```python
from build123d import *

# Parameters (mm, degrees)
SKETCH1_W            = 10
SKETCH1_H            = 50
SKETCH1_W_2          = 4
SKETCH1_H_2          = 30
BOSS_EXTRUDE1_DEPTH  = 2
SKETCH2_W            = 50
SKETCH2_H            = 10
SKETCH2_W_2          = 37
SKETCH2_H_2          = 5
BOSS_EXTRUDE2_DEPTH  = 12
SKETCH6_W            = 133.5
SKETCH6_H            = 10
SKETCH6_W_2          = 37
SKETCH6_H_2          = 5
BOSS_EXTRUDE7_DEPTH  = 2
SKETCH3_W            = 133.5
SKETCH3_H            = 10
BOSS_EXTRUDE3_DEPTH  = 5.7
SKETCH4_W            = 10.25
SKETCH4_H            = 10
BOSS_EXTRUDE4_DEPTH  = 10
CHAMFER1_SIZE        = 2
BOSS_EXTRUDE5_START  = -38
SKETCH5_W            = 10
SKETCH5_H            = 19
SKETCH5_R            = 2.2
BOSS_EXTRUDE5_DEPTH  = 2
BOSS_EXTRUDE6_START  = -24
SKETCH5_3_W          = 10
SKETCH5_3_H          = 22.4
SKETCH5_3_R          = 2
BOSS_EXTRUDE6_DEPTH  = 2
BOSS_EXTRUDE8_DEPTH  = 1
BOSS_EXTRUDE9_START  = -10
BOSS_EXTRUDE9_DEPTH  = 1
BOSS_EXTRUDE10_DEPTH = 1
BOSS_EXTRUDE11_START = -10
BOSS_EXTRUDE11_DEPTH = 1
BOSS_EXTRUDE12_START = -9.5
BOSS_EXTRUDE12_DEPTH = 10
BOSS_EXTRUDE13_DEPTH = 10
CHAMFER2_SIZE        = 10


with BuildPart() as part:
    # Sketch1 → Boss-Extrude1 (new body)
    with BuildSketch(Plane(origin=(0, 0, 0), x_dir=(0, 1, 0), z_dir=(0, 0, 1))):
        Rectangle(SKETCH1_W, SKETCH1_H)
        with Locations((-0.5, -3)):
            Rectangle(SKETCH1_W_2, SKETCH1_H_2, mode=Mode.SUBTRACT)
    extrude(amount=BOSS_EXTRUDE1_DEPTH)

    # Sketch2 → Boss-Extrude2 (add)
    with BuildSketch(Plane.XY.offset(2)):
        Rectangle(SKETCH2_W, SKETCH2_H)
        with Locations((3.5, -1)):
            Rectangle(SKETCH2_W_2, SKETCH2_H_2, mode=Mode.SUBTRACT)
    extrude(amount=BOSS_EXTRUDE2_DEPTH)

    # Sketch6 → Boss-Extrude7 (add)
    with BuildSketch(Plane.XY.offset(14)):
        with Locations((-41.75, 0)):
            Rectangle(SKETCH6_W, SKETCH6_H)
        with Locations((3.5, -1)):
            Rectangle(SKETCH6_W_2, SKETCH6_H_2, mode=Mode.SUBTRACT)
    extrude(amount=BOSS_EXTRUDE7_DEPTH)

    # Sketch3 → Boss-Extrude3 (add)
    with BuildSketch(Plane.XY.offset(16)):
        with Locations((-41.75, 0)):
            Rectangle(SKETCH3_W, SKETCH3_H)
        Polygon((22, -3.5), (-15, -3.5), (-15, -2), (-64.5, -2), (-64.5, 1.5), (22, 1.5), align=None, mode=Mode.SUBTRACT)
    extrude(amount=BOSS_EXTRUDE3_DEPTH)

    # Sketch4 → Boss-Extrude4 (add)
    with BuildSketch(Plane.XY.offset(21.7)):
        with Locations((-103.375, 0)):
            Rectangle(SKETCH4_W, SKETCH4_H)
        Polygon((-64.5, -2), (-64.5, 1.5), (-59.5, 1.5), (-59.5, 5), (-74.75, 5), (-74.75, -5), (25, -5), (25, 5), (1.7, 5), (1.7, 1.5), (22, 1.5), (22, -3.5), (-15, -3.5), (-15, -2), align=None)
    extrude(amount=BOSS_EXTRUDE4_DEPTH)

    # Chamfer1
    chamfer1_edges = [part.edges().sort_by_distance(p)[0] for p in [
        (-98.25, 0, 21.7),
        (-74.75, 0, 21.7),
    ]]
    chamfer(chamfer1_edges, length=CHAMFER1_SIZE)



with BuildPart() as body_2:
    # Sketch5 → Boss-Extrude5 (new body)
    with BuildSketch(Plane.XY.offset(31.7).offset(BOSS_EXTRUDE5_START)):
        with Locations((10.5, 14.5)):
            Rectangle(SKETCH5_W, SKETCH5_H)
        with Locations((10.5, 14.5)):
            Circle(SKETCH5_R, mode=Mode.SUBTRACT)
    extrude(amount=BOSS_EXTRUDE5_DEPTH)


with BuildPart() as body_3:
    # Sketch5<3> → Boss-Extrude6 (new body)
    with BuildSketch(Plane.XY.offset(31.7).offset(BOSS_EXTRUDE6_START)):
        with Locations((-103.5, 16.2)):
            Rectangle(SKETCH5_3_W, SKETCH5_3_H)
        with Locations((-103.5, 18.5)):
            Circle(SKETCH5_3_R, mode=Mode.SUBTRACT)
    extrude(amount=BOSS_EXTRUDE6_DEPTH)


with BuildPart() as part_1:
    add(part.part)

    add(body_2.part)  # Boss-Extrude8 merges body 2
    # Sketch7 → Boss-Extrude8 (add)
    with BuildSketch(Plane.YZ.offset(15.5)):
        Polygon((5, -4.3), (20, -4.3), (5, 7.7), align=None)
    extrude(amount=-BOSS_EXTRUDE8_DEPTH)

    # Sketch7<2> → Boss-Extrude9 (add)
    with BuildSketch(Plane.YZ.offset(15.5).offset(BOSS_EXTRUDE9_START)):
        Polygon((5, -4.3), (20, -4.3), (5, 7.7), align=None)
    extrude(amount=BOSS_EXTRUDE9_DEPTH)


    add(body_3.part)  # Boss-Extrude10 merges body 3
    # Sketch8 → Boss-Extrude10 (add)
    with BuildSketch(Plane.YZ.offset(-98.5)):
        Polygon((5, 9.7), (20, 9.7), (5, 21.7), align=None)
    extrude(amount=-BOSS_EXTRUDE10_DEPTH)

    # Sketch8<2> → Boss-Extrude11 (add)
    with BuildSketch(Plane.YZ.offset(-98.5).offset(BOSS_EXTRUDE11_START)):
        Polygon((5, 9.7), (20, 9.7), (5, 21.7), align=None)
    extrude(amount=BOSS_EXTRUDE11_DEPTH)

    # Sketch9 → Boss-Extrude12 (add)
    with BuildSketch(Plane.YZ.offset(25).offset(BOSS_EXTRUDE12_START)):
        Polygon((5, -6.3), (2, 0), (5, 0), align=None)
    extrude(amount=-BOSS_EXTRUDE12_DEPTH)

    # Sketch10 → Boss-Extrude13 (add)
    with BuildSketch(Plane.YZ.offset(-98.5)):
        Polygon((5, 7.7), (5, 14), (2, 14), align=None)
    extrude(amount=-BOSS_EXTRUDE13_DEPTH)

    # Chamfer2
    chamfer2_edges = [part_1.edges().sort_by_distance(p)[0] for p in [
        (-108.5, -5, 22.85),
    ]]
    chamfer(chamfer2_edges, length=CHAMFER2_SIZE)


solid = part_1.part
```
Design review of the part built by this model. Coordinates are the model's own, in mm. A direction names the side the tool comes from. Give positions to 0.01 mm unless a question says otherwise; leave off trailing zeros. Loops run counter-clockwise (first coordinate to the right, second up) from the corner with the lowest first, then second, coordinate; pieces in that order, holes last. Notation, with made-up numbers: M 51,3.25 L 70,3.25 A25 ccw 70,39.25 Z; hole C 62,-20 d6. An arc over 180 degrees is marked long. Return JSON: item names as keys, results as strings. Group by question number.
Item 1: We need section B-B (z = 12.5). Give the boundary of the cut face in (x, y), and give its area (3 significant figures).
Item 2: Insertion check: pin 1 Ø0.6 at (x, z) = (11, -5.5) entering from +Y; pin 2 Ø10 at (x, y) = (-66, 11.5) entering from -Z; pin 3 Ø15 at (x, z) = (6, 22) entering from +Y; pin 4 Ø8 at (x, y) = (-92, 5) entering from +Z. Each pin has a flat end and moves straight along its axis. Give the tip position at first contact, or say it passes through.
Item 3: For probe 1 along X at (y, z) = (7.5, 3.5); probe 2 along X at (y, z) = (-1, 12); probe 3 along Y at (x, z) = (-42, 17), list the stretches that pass through material, from the lowest coordinate up.
Item 4: We need section C-C (x = -103.5). Give the boundary of the cut face in (y, z).
Item 5: We need section A-A (y = 10). Give the boundary of the cut face in (x, z).
Item 6: We need section D-D (y = 18.5). Give the boundary of the cut face in (x, z).
Item 7: Mouldability with a two-part tool opening along X and no side actions: class faces 5 (the flat face through (-39, -2, 24)), 6 (the flat face through (-24, -5, 19)), 7 (the flat face through (-103.6, 0.1, 22.2)) as released by +X, released by -X, zero draft, split by the parting line, or undercut.
Item 8: Tool access review of faces 1 (the flat face through (-36.7, -2.2, 31.7)), 2 (the flat face through (-87, 0, 21.7)), 3 (the flat face through (3, -3, 2)), 4 (the flat face through (-107.5, 9, 13)): name each direction out of +Z, -Z, +X, -X, +Y, -Y from which nothing blocks a thin tool from reaching the whole face with its end or side.
Output:
{
 "1": {"outline": "M -108.5,5 L -106.21,2.71 L -98.5,2.71 L -98.5,16.5 L -99.5,16.5 L -99.5,5 L -107.5,5 L -107.5,16.5 L -108.5,16.5 Z; M -25,-5 L 25,-5 L 25,5 L -25,5 Z; hole M -15,-3.5 L 22,-3.5 L 22,1.5 L -15,1.5 Z", "area": "358 mm^2"},
 "2": {"pin 1": "stops at y = 24", "pin 2": "passes through", "pin 3": "stops at y = 5", "pin 4": "stops at z = 21.7"},
 "3": {"probe 1": "x = 5.5 to 6.5, 14.5 to 15.5", "probe 2": "x = -25 to -15, 22 to 25", "probe 3": "y = -5 to -2, 1.5 to 5"},
 "4": {"outline": "M 0,14 L 2,14 L 5,7.7 L 16.5,7.7 L 16.5,9.7 L 5,9.7 L 5,31.7 L 0,31.7 Z; M 20.5,7.7 L 27.4,7.7 L 27.4,9.7 L 20.5,9.7 Z"},
 "5": {"outline": "M -108.5,7.7 L -98.5,7.7 L -98.5,17.7 L -99.5,17.7 L -99.5,9.7 L -107.5,9.7 L -107.5,17.7 L -108.5,17.7 Z; M 5.5,-6.3 L 15.5,-6.3 L 15.5,3.7 L 14.5,3.7 L 14.5,-4.3 L 6.5,-4.3 L 6.5,3.7 L 5.5,3.7 Z"},
 "6": {"outline": "M -108.5,7.7 L -105.5,7.7 L -105.5,9.7 L -107.5,9.7 L -107.5,10.9 L -108.5,10.9 Z; M -101.5,7.7 L -98.5,7.7 L -98.5,10.9 L -99.5,10.9 L -99.5,9.7 L -101.5,9.7 Z; M 5.5,-6.3 L 15.5,-6.3 L 15.5,-3.1 L 14.5,-3.1 L 14.5,-4.3 L 6.5,-4.3 L 6.5,-3.1 L 5.5,-3.1 Z"},
 "7": {"face 5": "undercut", "face 6": "zero draft", "face 7": "released by -X"},
 "8": {"face 1": "+Z, +X, -X, +Y, -Y", "face 2": "+Z, +Y, -Y", "face 3": "+Z", "face 4": "+Z, +Y"}
}
